Work out the finished part from the listing and answer in its coordinate system (mm). Face numbers are marked on the shaded views. A direction names the side the tool comes from. Coordinates: 2 decimals unless noted, no trailing zeros. Write each loop counter-clockwise with the first axis right and the second up, starting at its lowest first coordinate (ties: lowest second). Pieces come first, ordered by that corner, then holes. Notation, with made-up numbers: (32, 41) - (41, 41) arc R18 ccw to (41, 72) - close; hole circle Ø5 at (-22.75, -5). An arc over 180 degrees is marked (long way). Use one line per item in the form item = value. Start each with the question number.
Item 1: A cutting plane is placed at A-A (y = 0). Write down the section's boundary in (x, z).
Item 2: A cutting plane is placed at D-D (z = -3.25). Write down the section's boundary in (x, y).
Item 3: Consider probe 1 along Z at (x, y) = (6.5, 0); probe 2 along X at (y, z) = (-4, 0.25); probe 3 along Y at (x, z) = (8, 1). Determine where each line is inside the solid, lowest interval first.
Item 4: Given pin 1 (6 mm diameter, centred on y = 4, z = 3.5, fed in from -X); pin 2 (1.5 mm diameter, centred on y = 3.5, z = -2.5, fed in from +X); pin 3 (1.5 mm diameter, centred on x = 6.5, z = 1, fed in from +Y), each flat-ended and moving along its own axis, determine where each tip first touches the part or whether it passes through.
Item 5: For the marked faces 1 and 2, determine the directions among +Z, -Z, +X, -X, +Y, -Y from which every point of the face is accessible in a straight line to the end or side of a thin tool.
Item 6: A cutting plane is placed at C-C (x = 8). Write down the section's boundary in (y, z), then the cut area to 3 significant figures.
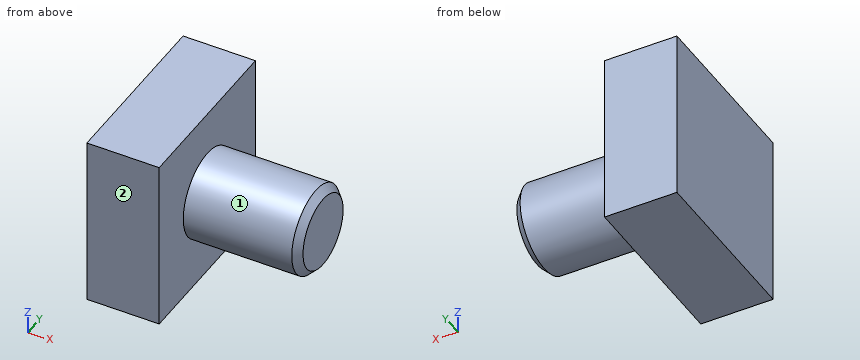
from build123d import *

# Parameters (mm, degrees)
F0_W     = 12
F0_H     = 12
F1_DEPTH = 5
F2_R     = 3
F3_DEPTH = 8
F4_SIZE  = 0.5


with BuildPart() as f1:
    # F0 (on Right) → F1 (new body)
    with BuildSketch(Plane.YZ):
        Rectangle(F0_W, F0_H)
    extrude(amount=F1_DEPTH)

    # F2 (on face) → F3 (join)
    with BuildSketch(Plane.YZ.offset(5)):
        Circle(F2_R)
    extrude(amount=F3_DEPTH)

    # F4
    f4_edges = [f1.edges().sort_by_distance(p)[0] for p in [
        (13, -3, 0),
    ]]
    chamfer(f4_edges, length=F4_SIZE)


solid = f1.part
Answer:
q1.outline = (0, -6) - (5, -6) - (5, -3) - (12.5, -3) - (13, -2.5) - (13, 2.5) - (12.5, 3) - (5, 3) - (5, 6) - (0, 6) - close
q2.outline = (0, -6) - (5, -6) - (5, 6) - (0, 6) - close
q3.probe_1 = -3 to 3
q3.probe_2 = 0 to 5
q3.probe_3 = -2.83 to 2.83
q4.pin_1 = 0
q4.pin_2 = 5
q4.pin_3 = 2.99
q5.face_1 = +X
q5.face_2 = +Z, -Z, +X, -X, -Y
q6.outline = circle Ø6 at (0, 0)
q6.area = 28.3 mm²
